Design review of the part built by this model. Coordinates are the model's own, in mm. Face numbers are marked on the shaded views. A direction names the side the tool comes from. Give positions to 0.01 mm unless a question says otherwise; leave off trailing zeros. Write each loop counter-clockwise with the first axis right and the second up, starting at its lowest first coordinate (ties: lowest second). Pieces come first, ordered by that corner, then holes. Notation, with made-up numbers: (14, 27) -> (30, 27) arc R34 cw to (30, 65) -> close; hole circle Ø6 at (-11, -27). An arc over 180 degrees is marked (long way). Use CSV: the item, a comma, the result in double quotes.
```python
from build123d import *

# Parameters (mm, degrees)
SKETCH1_W           = 32
SKETCH1_H           = 48
BOSS_EXTRUDE1_DEPTH = 0.5
BOSS_EXTRUDE2_DEPTH = 1
SKETCH3_W           = 36
SKETCH3_H           = 11.5
BOSS_EXTRUDE3_DEPTH = 0.3


with BuildPart() as part:
    # Sketch1 → Boss-Extrude1 (new body)
    with BuildSketch(Plane(origin=(0, 0, 0), x_dir=(1, 0, 0), z_dir=(0, 1, 0))):
        Rectangle(SKETCH1_W, SKETCH1_H)
    extrude(amount=BOSS_EXTRUDE1_DEPTH)

    # Sketch2 → Boss-Extrude2 (add)
    with BuildSketch(Plane(origin=(0, 0.5, 0), x_dir=(1, 0, 0), z_dir=(0, 1, 0))):
        with BuildLine():
            Line((-5.744434592, 22.704745015), (2.282363543, 22.704745015))
            ThreePointArc((2.282363543, 22.704745015), (7.585664402, 20.508045873), (9.782363543, 15.204745015))
            Line((9.782363543, 15.204745015), (9.782363543, -2.322620184))
            ThreePointArc((9.782363543, -2.322620184), (7.585664402, -7.625921042), (2.282363543, -9.822620184))
            Line((2.282363543, -9.822620184), (-5.744434592, -9.822620184))
            ThreePointArc((-5.744434592, -9.822620184), (-11.047735451, -7.625921042), (-13.244434592, -2.322620184))
            Line((-13.244434592, -2.322620184), (-13.244434592, 15.204745015))
            ThreePointArc((-13.244434592, 15.204745015), (-11.047735451, 20.508045873), (-5.744434592, 22.704745015))
        make_face()
        with BuildLine():
            Line((-4.515159693, 14.894956836), (1.133601925, 14.894956836))
            ThreePointArc((1.133601925, 14.894956836), (1.840708706, 14.602063617), (2.133601925, 13.894956836))
            Line((2.133601925, 13.894956836), (2.133601925, -1.334885126))
            ThreePointArc((2.133601925, -1.334885126), (1.840708706, -2.041991907), (1.133601925, -2.334885126))
            Line((1.133601925, -2.334885126), (-4.515159693, -2.334885126))
            ThreePointArc((-4.515159693, -2.334885126), (-5.222266474, -2.041991907), (-5.515159693, -1.334885126))
            Line((-5.515159693, -1.334885126), (-5.515159693, 13.894956836))
            ThreePointArc((-5.515159693, 13.894956836), (-5.222266474, 14.602063617), (-4.515159693, 14.894956836))
        make_face(mode=Mode.SUBTRACT)
    extrude(amount=BOSS_EXTRUDE2_DEPTH)

    # Sketch3 → Boss-Extrude3 (add)
    with BuildSketch(Plane.XZ):
        with Locations((-2, 18.25)):
            Rectangle(SKETCH3_W, SKETCH3_H)
    extrude(amount=BOSS_EXTRUDE3_DEPTH)


solid = part.part
```
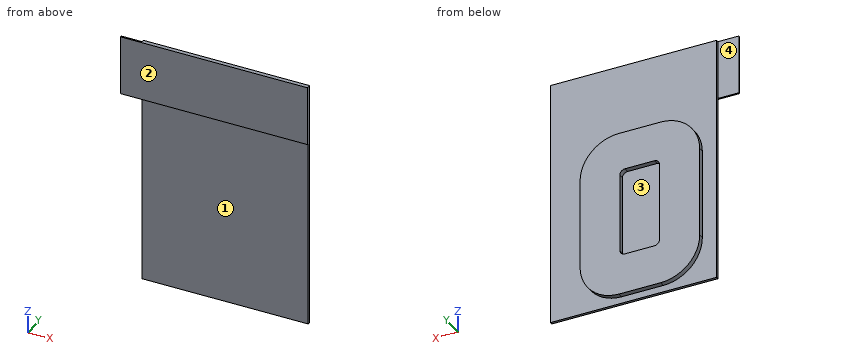
(1) Take a section at B-B (z = -3). Write out the cut boundary in (x, y), then the cut area to 3 significant figures.
Established:
outline,"(-16, 0) -> (16, 0) -> (16, 0.5) -> (9.78, 0.5) -> (9.78, 1.5) -> (2.13, 1.5) -> (2.13, 0.5) -> (-5.52, 0.5) -> (-5.52, 1.5) -> (-13.24, 1.5) -> (-13.24, 0.5) -> (-16, 0.5) -> close"
area,"31.4 mm2"
(2) Mouldability with a two-part tool opening along Z and no side actions: class the marked faces 3 and 4 as +Z half, -Z half, draft (parallel to the pull), parting line (faces both ways), or undercut.
Established:
face 3,"undercut"
face 4,"draft"
(3) Take a section at A-A (y = 1.05). Write out the cut boundary in (x, z), then the cut area to 3 significant figures.
Established:
outline,"(-13.24, -15.2) arc R7.5 ccw to (-5.74, -22.7) -> (2.28, -22.7) arc R7.5 ccw to (9.78, -15.2) -> (9.78, 2.32) arc R7.5 ccw to (2.28, 9.82) -> (-5.74, 9.82) arc R7.5 ccw to (-13.24, 2.32) -> close; hole (-5.52, -13.89) arc R1 ccw to (-4.52, -14.89) -> (1.13, -14.89) arc R1 ccw to (2.13, -13.89) -> (2.13, 1.33) arc R1 ccw to (1.13, 2.33) -> (-4.52, 2.33) arc R1 ccw to (-5.52, 1.33) -> close"
area,"570 mm2"
(4) Take a section at D-D (z = -18.5). Write out the cut boundary in (x, y).
Established:
outline,"(-16, 0) -> (16, 0) -> (16, 0.5) -> (9.02, 0.5) -> (9.02, 1.5) -> (-12.48, 1.5) -> (-12.48, 0.5) -> (-16, 0.5) -> close"
(5) Tool access review of the marked faces 1 and 2: name each direction out of +Z, -Z, +X, -X, +Y, -Y from which nothing blocks a thin tool from reaching the whole face with its end or side.
Established:
face 1,"-Z, +X, -X, -Y"
face 2,"+Z, -Z, +X, -X, -Y"
(6) Clearance check with flat-ended pins moving along their axes: pin 1 (16 mm diameter, centred on x = 0.5, z = -13.5, fed in from -Y); pin 2 (3 mm diameter, centred on x = -18, z = 20.5, fed in from +Y); pin 3 (4 mm diameter, centred on x = -2, z = -9.5, fed in from +Y). State where each tip first meets the part, or that it passes through.
Established:
pin 1,"stops at y = 0"
pin 2,"stops at y = 0"
pin 3,"stops at y = 0.5"
(7) For line 1 along Y through (x, z) = (4.5, -1); line 2 along Y through (x, z) = (0.5, -10); line 3 along X through (y, z) = (0.9, -10), list the stretches that pass through material, from the lowest coordinate up. Write a range as [from, to].
Established:
line 1,"y = [0, 1.5]"
line 2,"y = [0, 0.5]"
line 3,"x = [-13.24, -5.52], [2.13, 9.78]"
(8) Take a section at C-C (x = 0.5). Write out the cut boundary in (y, z).
Established:
outline,"(-0.3, 12.5) -> (0, 12.5) -> (0, -24) -> (0.5, -24) -> (0.5, -22.7) -> (1.5, -22.7) -> (1.5, -14.89) -> (0.5, -14.89) -> (0.5, 2.33) -> (1.5, 2.33) -> (1.5, 9.82) -> (0.5, 9.82) -> (0.5, 24) -> (-0.3, 24) -> close"
